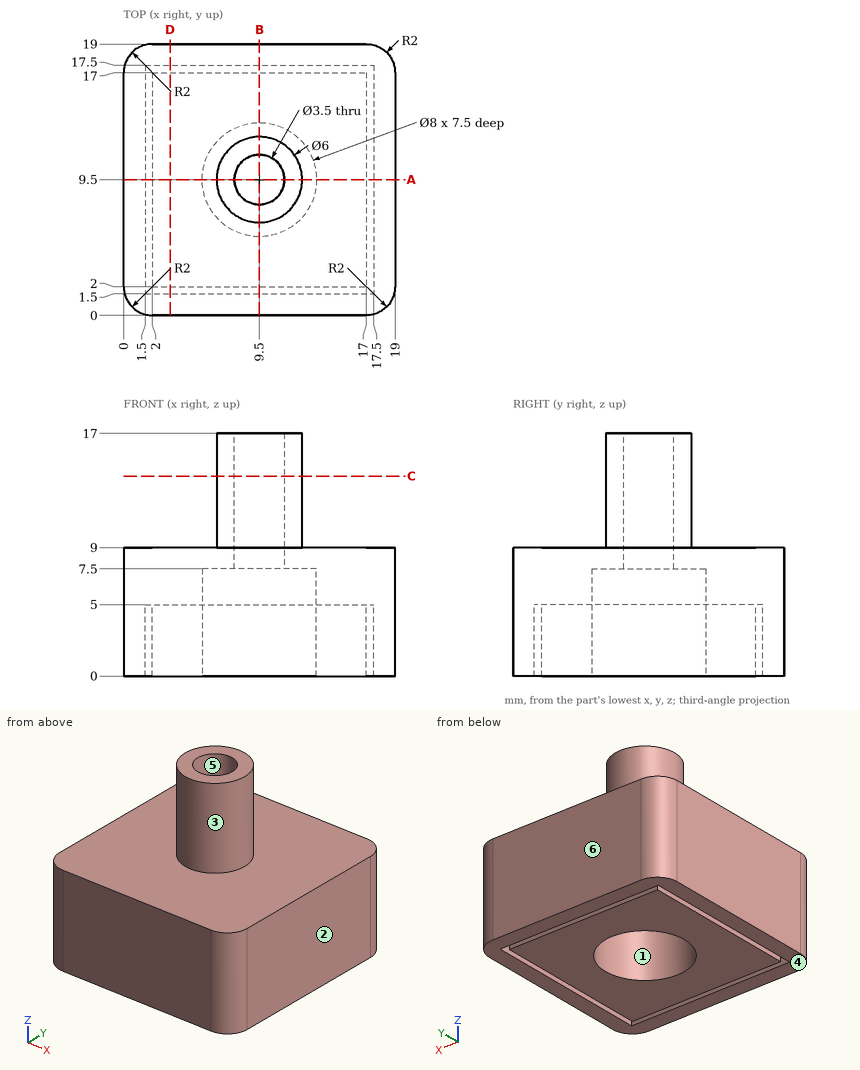
Print and shaded views of the part. All mm, measured from the part's lowest x, y and z. A direction names the side the tool comes from. Give positions to 0.01 mm unless a question says otherwise; leave off trailing zeros. Order: outer loops, then holes, each group sorted by start corner. A loop starts at its lowest first (then second) coordinate and runs counter-clockwise, first axis right, second up. Notation, with made-up numbers: M 28.25,-2.75 L 63.25,-2.75 A31 cw 63.25,32.25 Z; hole C -29.5,89 d2. An arc over 180 degrees is marked long. Use one line per item in the form item = value.
Q1. Wall check: probe 1 along X at (y, z) = (9.5, 3); probe 2 along Y at (x, z) = (9.5, 10). Give the ranges that are in metal, low to high.
Conclusion:
probe_1 = 0 to 1.5, 2 to 5.5, 13.5 to 17, 17.5 to 19
probe_2 = 6.5 to 7.75, 11.25 to 12.5
Q2. Slice it at C-C, the plane z = 14. Write the cut outline in (x, y), and give its area (3 significant figures).
Conclusion:
outline = C 9.5,9.5 d6; hole C 9.5,9.5 d3.5
area = 18.7 mm2
Q3. Pin check, flat tips, straight feed: P1, Ø10, axis at x = 10, z = 15, coming from the -Y side; P2, Ø4, axis at x = 9.5, y = 9.5, coming from the -Z side; P3, Ø8, axis at y = 3.5, z = 14, coming from the -X side. Stop position of each tip, or through.
Conclusion:
P1 = 6.5
P2 = 7.5
P3 = 7.26
Q4. Slice it at D-D, the plane x = 3.25. Write the cut outline in (y, z), and give its area (3 significant figures).
Conclusion:
outline = M 0,0 L 1.5,0 L 1.5,5 L 2,5 L 2,0 L 17,0 L 17,5 L 17.5,5 L 17.5,0 L 19,0 L 19,9 L 0,9 Z
area = 166 mm2
Q5. Which spindle directions (+Z, -Z, +X, -X, +Y, -Y) get a long thin tool onto all of the face, cutting with end or side? Do the marked faces 1, 2 and 3. Say none if no direction does.
Conclusion:
face_1 = -Z
face_2 = +Z, -Z, +X, +Y, -Y
face_3 = +Z
Q6. Pull direction Y, two halves, no side cores. Call the marked faces 4, 5 and 6: released by +Y, released by -Y, zero draft, split by the parting line, or undercut.
Conclusion:
face_4 = zero draft
face_5 = undercut
face_6 = released by +Y
Q7. Slice it at A-A, the plane y = 9.5. Write the cut outline in (x, z).
Conclusion:
outline = M 0,0 L 1.5,0 L 1.5,5 L 2,5 L 2,0 L 5.5,0 L 5.5,7.5 L 7.75,7.5 L 7.75,17 L 6.5,17 L 6.5,9 L 0,9 Z; M 11.25,7.5 L 13.5,7.5 L 13.5,0 L 17,0 L 17,5 L 17.5,5 L 17.5,0 L 19,0 L 19,9 L 12.5,9 L 12.5,17 L 11.25,17 Z
